Build history of the part. All positions in model axes, mm. Face numbers are marked on the shaded views. A direction names the side the tool comes from. Coordinates: 2 decimals unless noted, no trailing zeros. Loops run counter-clockwise (first coordinate to the right, second up) from the corner with the lowest first, then second, coordinate; pieces in that order, holes last.
(1) Wall check: L1, parallel to Z at x = -2.25, y = -0.5; L2, parallel to Y at x = 0.5, z = 3; L3, parallel to Y at x = -0.75, z = -3.5. Give the ranges that are in metal, low to high.
(2) Flat gauge pins, fed straight in: P1, Ø2, axis at x = -3.5, z = 0.5, coming from the +Y side; P2, Ø0.7, axis at y = -1.5, z = -1.5, coming from the +X side; P3, Ø0.7, axis at x = -0.5, z = 3, coming from the -Y side. Where does each tip first touch, or does it go through?
(3) Slice it at C-C (y = 0.5). Give the cut face in (x, z).
(4) Two-plate mould, pull along X, no slides. Class the marked faces 1, 2, 3 and 4: pulls with the +X half, pulls with the -X half, needs draft (parallel to the pull), parting line crosses it, or undercut.
(5) Tool access for the marked faces 5, 6 and 7: list every direction of +Z, -Z, +X, -X, +Y, -Y with a clear straight run to the whole face (end or side of a thin tool).
(6) Slice it at B-B (z = 1). Give the cut face in (x, y).
(7) Slice it at A-A (x = 0). Give the cut face in (y, z), and give its area (3 significant figures).
from build123d import *

# Parameters (mm, degrees)
SKETCH1_R           = 5
SKETCH1_R_2         = 2.400014974
BOSS_EXTRUDE1_DEPTH = 5
BOSS_EXTRUDE2_START = -5
SKETCH1_5_R         = 5
SKETCH1_5_R_2       = 2.400014974
BOSS_EXTRUDE2_DEPTH = 5


with BuildPart() as part:
    # Sketch1 → Boss-Extrude1 (new body)
    # profile 1 of 12: a face of its own
    with BuildSketch(Plane.XY):
        Circle(SKETCH1_R)
        Circle(SKETCH1_R_2, mode=Mode.SUBTRACT)
    # profile 2 of 12: a face of its own
    with BuildSketch(Plane.XY):
        with BuildLine():
            ThreePointArc((-0.799911499, -1.268913549), (-1.060590017, -1.060730322), (-1.268807724, -0.800079346))
            Line((-1.268807724, -0.800079346), (-2.262729528, -0.800079346))
            ThreePointArc((-2.262729528, -0.800079346), (-1.69700392, -1.697129804), (-0.799911499, -2.26278887))
            Line((-0.799911499, -2.26278887), (-0.799911499, -1.268913549))
        make_face()
    # profile 3 of 12: a face of its own
    with BuildSketch(Plane.XY):
        with BuildLine():
            ThreePointArc((0.800079346, -1.268807724), (9.9211e-05, -1.499999997), (-0.799911499, -1.268913549))
            Line((-0.799911499, -1.268913549), (-0.799911499, -2.26278887))
            ThreePointArc((-0.799911499, -2.26278887), (8.9014e-05, -2.400014973), (0.800079346, -2.262729528))
            Line((0.800079346, -2.262729528), (0.800079346, -1.268807724))
        make_face()
    # profile 4 of 12: a face of its own
    with BuildSketch(Plane.XY):
        with BuildLine():
            ThreePointArc((-1.268807724, -0.800079346), (-1.499999997, -9.9211e-05), (-1.268913549, 0.799911499))
            Line((-1.268913549, 0.799911499), (-2.26278887, 0.799911499))
            ThreePointArc((-2.26278887, 0.799911499), (-2.400014973, -8.9014e-05), (-2.262729528, -0.800079346))
            Line((-2.262729528, -0.800079346), (-1.268807724, -0.800079346))
        make_face()
    # profile 5 of 12: a face of its own
    with BuildSketch(Plane.XY):
        with BuildLine():
            ThreePointArc((-1.268913549, 0.799911499), (-1.197659588, 0.903112126), (-1.118033989, 1))
            ThreePointArc((-1.118033989, 1), (-0.96842867, 1.145489376), (-0.800079346, 1.268807724))
            Line((-0.800079346, 1.268807724), (-0.800079346, 2.262729528))
            ThreePointArc((-0.800079346, 2.262729528), (-1.697129804, 1.69700392), (-2.26278887, 0.799911499))
            Line((-2.26278887, 0.799911499), (-1.268913549, 0.799911499))
        make_face()
    # profile 6 of 12: a face of its own
    with BuildSketch(Plane.XY):
        with BuildLine():
            Line((-0.800079346, 2.262729528), (-0.800079346, 1.268807724))
            ThreePointArc((-0.800079346, 1.268807724), (-9.9211e-05, 1.499999997), (0.799911499, 1.268913549))
            Line((0.799911499, 1.268913549), (0.799911499, 2.26278887))
            ThreePointArc((0.799911499, 2.26278887), (-8.9014e-05, 2.400014973), (-0.800079346, 2.262729528))
        make_face()
    # profile 7 of 12: a face of its own
    with BuildSketch(Plane.XY):
        with BuildLine():
            Line((0.799911499, 2.26278887), (0.799911499, 1.268913549))
            ThreePointArc((0.799911499, 1.268913549), (0.968352905, 1.145553426), (1.118033989, 1))
            ThreePointArc((1.118033989, 1), (1.197599853, 0.903191338), (1.268807724, 0.800079346))
            Line((1.268807724, 0.800079346), (2.262729528, 0.800079346))
            ThreePointArc((2.262729528, 0.800079346), (1.69700392, 1.697129804), (0.799911499, 2.26278887))
        make_face()
    # profile 8 of 12: a face of its own
    with BuildSketch(Plane.XY):
        with BuildLine():
            Line((2.262729528, 0.800079346), (1.268807724, 0.800079346))
            ThreePointArc((1.268807724, 0.800079346), (1.4410433, 0.4164063), (1.5, 0))
            ThreePointArc((1.5, 0), (1.441070838, -0.416310988), (1.268913549, -0.799911499))
            Line((1.268913549, -0.799911499), (2.26278887, -0.799911499))
            ThreePointArc((2.26278887, -0.799911499), (2.365459685, -0.405798414), (2.400014974, 0))
            ThreePointArc((2.400014974, 0), (2.365444633, 0.405886146), (2.262729528, 0.800079346))
        make_face()
    # profile 9 of 12: a face of its own
    with BuildSketch(Plane.XY):
        with BuildLine():
            ThreePointArc((1.268913549, -0.799911499), (1.060730322, -1.060590017), (0.800079346, -1.268807724))
            Line((0.800079346, -1.268807724), (0.800079346, -2.262729528))
            ThreePointArc((0.800079346, -2.262729528), (1.697129804, -1.69700392), (2.26278887, -0.799911499))
            Line((2.26278887, -0.799911499), (1.268913549, -0.799911499))
        make_face()
    # profile 10 of 12: a face of its own
    with BuildSketch(Plane.XY):
        with BuildLine():
            Line((-0.800079346, 1.268807724), (-0.800079346, 1))
            Line((-0.800079346, 1), (0.799911499, 1))
            Line((0.799911499, 1), (0.799911499, 1.268913549))
            ThreePointArc((0.799911499, 1.268913549), (-9.9211e-05, 1.499999997), (-0.800079346, 1.268807724))
        make_face()
    # profile 11 of 12: a face of its own
    with BuildSketch(Plane.XY):
        with BuildLine():
            Line((0.799911499, 1.268913549), (0.799911499, 1))
            Line((0.799911499, 1), (1.118033989, 1))
            ThreePointArc((1.118033989, 1), (0.968352905, 1.145553426), (0.799911499, 1.268913549))
        make_face()
    # profile 12 of 12: a face of its own
    with BuildSketch(Plane.XY):
        with BuildLine():
            ThreePointArc((-0.800079346, 1.268807724), (-0.96842867, 1.145489376), (-1.118033989, 1))
            Line((-1.118033989, 1), (-0.800079346, 1))
            Line((-0.800079346, 1), (-0.800079346, 1.268807724))
        make_face()
    extrude(amount=BOSS_EXTRUDE1_DEPTH)

    # Sketch1<5> → Boss-Extrude2 (add)
    # profile 1 of 11: a face of its own
    with BuildSketch(Plane.XY.offset(BOSS_EXTRUDE2_START)):
        Circle(SKETCH1_5_R)
        Circle(SKETCH1_5_R_2, mode=Mode.SUBTRACT)
    # profile 2 of 11: a face of its own
    with BuildSketch(Plane.XY.offset(BOSS_EXTRUDE2_START)):
        with BuildLine():
            ThreePointArc((1.268913549, -0.799911499), (1.060730322, -1.060590017), (0.800079346, -1.268807724))
            Line((0.800079346, -1.268807724), (0.800079346, -2.262729528))
            ThreePointArc((0.800079346, -2.262729528), (1.697129804, -1.69700392), (2.26278887, -0.799911499))
            Line((2.26278887, -0.799911499), (1.268913549, -0.799911499))
        make_face()
    # profile 3 of 11: a face of its own
    with BuildSketch(Plane.XY.offset(BOSS_EXTRUDE2_START)):
        with BuildLine():
            Line((0.799911499, 2.26278887), (0.799911499, 1.268913549))
            ThreePointArc((0.799911499, 1.268913549), (0.968352905, 1.145553426), (1.118033989, 1))
            ThreePointArc((1.118033989, 1), (1.197599853, 0.903191338), (1.268807724, 0.800079346))
            Line((1.268807724, 0.800079346), (2.262729528, 0.800079346))
            ThreePointArc((2.262729528, 0.800079346), (1.69700392, 1.697129804), (0.799911499, 2.26278887))
        make_face()
    # profile 4 of 11: a face of its own
    with BuildSketch(Plane.XY.offset(BOSS_EXTRUDE2_START)):
        with BuildLine():
            ThreePointArc((-1.268913549, 0.799911499), (-1.197659588, 0.903112126), (-1.118033989, 1))
            ThreePointArc((-1.118033989, 1), (-0.96842867, 1.145489376), (-0.800079346, 1.268807724))
            Line((-0.800079346, 1.268807724), (-0.800079346, 2.262729528))
            ThreePointArc((-0.800079346, 2.262729528), (-1.697129804, 1.69700392), (-2.26278887, 0.799911499))
            Line((-2.26278887, 0.799911499), (-1.268913549, 0.799911499))
        make_face()
    # profile 5 of 11: a face of its own
    with BuildSketch(Plane.XY.offset(BOSS_EXTRUDE2_START)):
        with BuildLine():
            ThreePointArc((-0.799911499, -1.268913549), (-1.060590017, -1.060730322), (-1.268807724, -0.800079346))
            Line((-1.268807724, -0.800079346), (-2.262729528, -0.800079346))
            ThreePointArc((-2.262729528, -0.800079346), (-1.69700392, -1.697129804), (-0.799911499, -2.26278887))
            Line((-0.799911499, -2.26278887), (-0.799911499, -1.268913549))
        make_face()
    # profile 6 of 11: a face of its own
    with BuildSketch(Plane.XY.offset(BOSS_EXTRUDE2_START)):
        with BuildLine():
            Line((0.799911499, 1.268913549), (0.799911499, 1))
            Line((0.799911499, 1), (1.118033989, 1))
            ThreePointArc((1.118033989, 1), (0.968352905, 1.145553426), (0.799911499, 1.268913549))
        make_face()
    # profile 7 of 11: a face of its own
    with BuildSketch(Plane.XY.offset(BOSS_EXTRUDE2_START)):
        with BuildLine():
            ThreePointArc((-0.800079346, 1.268807724), (-0.96842867, 1.145489376), (-1.118033989, 1))
            Line((-1.118033989, 1), (-0.800079346, 1))
            Line((-0.800079346, 1), (-0.800079346, 1.268807724))
        make_face()
    # profile 8 of 11: a face of its own
    with BuildSketch(Plane.XY.offset(BOSS_EXTRUDE2_START)):
        with BuildLine():
            Line((-0.800079346, 1), (-1.118033989, 1))
            ThreePointArc((-1.118033989, 1), (-1.197659588, 0.903112126), (-1.268913549, 0.799911499))
            Line((-1.268913549, 0.799911499), (-0.800017929, 0.799911499))
            Line((-0.800017929, 0.799911499), (-0.800079346, 0.800017929))
            Line((-0.800079346, 0.800017929), (-0.800079346, 1))
        make_face()
    # profile 9 of 11: a face of its own
    with BuildSketch(Plane.XY.offset(BOSS_EXTRUDE2_START)):
        with BuildLine():
            Line((1.118033989, 1), (0.799911499, 1))
            Line((0.799911499, 1), (0.799911499, 0.800017929))
            Line((0.799911499, 0.800017929), (0.800017929, 0.800079346))
            Line((0.800017929, 0.800079346), (1.268807724, 0.800079346))
            ThreePointArc((1.268807724, 0.800079346), (1.197599853, 0.903191338), (1.118033989, 1))
        make_face()
    # profile 10 of 11: a face of its own
    with BuildSketch(Plane.XY.offset(BOSS_EXTRUDE2_START)):
        with BuildLine():
            Line((0.800079346, -0.800017929), (0.800079346, -1.268807724))
            ThreePointArc((0.800079346, -1.268807724), (1.060730322, -1.060590017), (1.268913549, -0.799911499))
            Line((1.268913549, -0.799911499), (0.800017929, -0.799911499))
            Line((0.800017929, -0.799911499), (0.800079346, -0.800017929))
        make_face()
    # profile 11 of 11: a face of its own
    with BuildSketch(Plane.XY.offset(BOSS_EXTRUDE2_START)):
        with BuildLine():
            Line((-0.800017929, -0.800079346), (-1.268807724, -0.800079346))
            ThreePointArc((-1.268807724, -0.800079346), (-1.060590017, -1.060730322), (-0.799911499, -1.268913549))
            Line((-0.799911499, -1.268913549), (-0.799911499, -0.800017929))
            Line((-0.799911499, -0.800017929), (-0.800017929, -0.800079346))
        make_face()
    extrude(amount=BOSS_EXTRUDE2_DEPTH)


solid = part.part
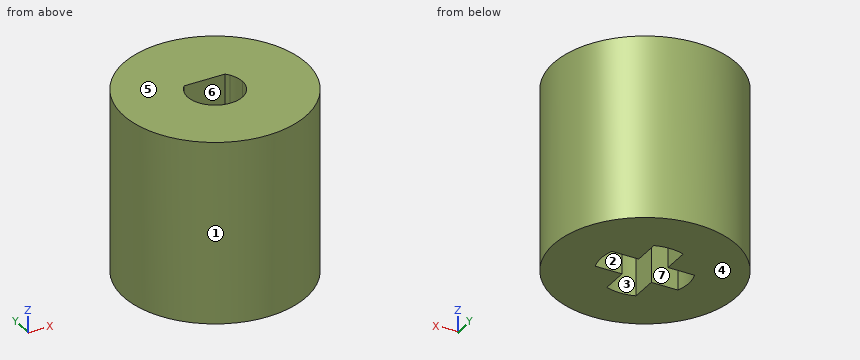
Response values:
1. L1: z = 0 to 5
1. L2: y = -4.97 to -1.41, 1 to 4.97
1. L3: y = -4.94 to -2.28, 2.28 to 4.94
2. P1: stops at y = 4.33
2. P2: stops at x = 4.87
2. P3: stops at y = -5
3. outline: (-4.97, -5) - (-2.35, -5) - (-2.35, 0) - (-1.41, 0) - (-1.41, 5) - (-4.97, 5) - close; (1.41, 0) - (2.35, 0) - (2.35, -5) - (4.97, -5) - (4.97, 5) - (1.41, 5) - close
4. face 1: parting line crosses it
4. face 2: undercut
4. face 3: undercut
4. face 4: needs draft
5. face 5: +Z, +X, -X, +Y, -Y
5. face 6: +Z
5. face 7: -Z
6. outline: circle Ø10 at (0, 0); hole (-1.12, 1) arc R1.5 ccw (long way) to (1.12, 1) - close
7. outline: (-5, -5) - (-2.4, -5) - (-2.4, 0) - (-1.5, 0) - (-1.5, 5) - (-5, 5) - close; (1, 0) - (2.4, 0) - (2.4, -5) - (5, -5) - (5, 5) - (1, 5) - close
7. area: 63.5 mm2
